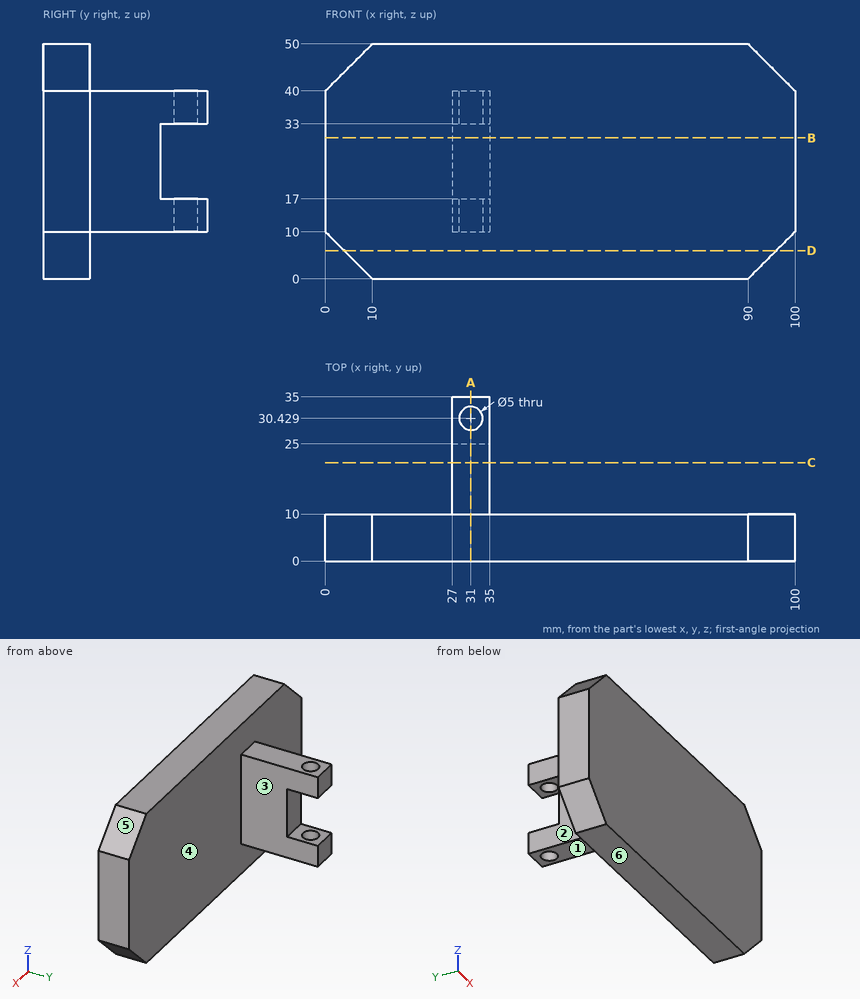
Drawing for the job (mm, zero at the part's lowest x, y, z). A direction names the side the tool comes from. Give positions to 0.01 mm unless a question says otherwise; leave off trailing zeros. Order: outer loops, then holes, each group sorted by start corner. A loop starts at its lowest first (then second) coordinate and runs counter-clockwise, first axis right, second up. Notation, with made-up numbers: M -33.5,70 L -5.5,70 A27 ccw -5.5,103 Z; hole C -28,23.25 d9. An arc over 180 degrees is marked long. Put each result on its own line as item: value. Start each with the question number.
(1) Saw through at A-A, the plane x = 31. Write the cut outline in (y, z).
(2) Saw through at D-D, the plane z = 6. Write the cut outline in (x, y).
(3) Saw through at C-C, the plane y = 21. Write the cut outline in (x, z).
(4) Mould opens along Z. For the marked faces 4, 5 and 6 say: +Z half, -Z half, draft (parallel to the pull), parting line (faces both ways), or undercut.
(5) Which spindle directions (+Z, -Z, +X, -X, +Y, -Y) get a long thin tool onto all of the face, cutting with end or side? Do the marked faces 1, 2 and 3. Say none if no direction does.
(6) Saw through at B-B, the plane z = 30. Write the cut outline in (x, y), then the cut area to 3 significant figures.
(7) Flat gauge pins, fed straight in: pin 1 Ø6 at (y, z) = (14, 37.5) entering from +X; pin 2 Ø6.5 at (x, y) = (30, 23.5) entering from -Z; pin 3 Ø9 at (x, y) = (32.5, 29) entering from +Z; pin 4 Ø5 at (y, z) = (16.5, 5.5) entering from +X. Where does each tip first touch, or does it go through?
(8) Drill centre lines: line 1 along Y through (x, z) = (31, 35); line 2 along X through (y, z) = (27, 14); line 3 along Z through (x, y) = (33, 19). Where is each one in solid material? Low to high.
Check result:
1. outline: M 0,0 L 10,0 L 10,10 L 27.93,10 L 27.93,17 L 25,17 L 25,33 L 27.93,33 L 27.93,40 L 10,40 L 10,50 L 0,50 Z; M 32.93,10 L 35,10 L 35,17 L 32.93,17 Z; M 32.93,33 L 35,33 L 35,40 L 32.93,40 Z
2. outline: M 4,0 L 96,0 L 96,10 L 4,10 Z
3. outline: M 27,10 L 35,10 L 35,40 L 27,40 Z
4. face 4: draft
4. face 5: +Z half
4. face 6: -Z half
5. face 1: -Z, +X, -X, +Y
5. face 2: +Z, -Z, -X, +Y
5. face 3: +Z, -Z, +X, +Y
6. outline: M 0,0 L 100,0 L 100,10 L 35,10 L 35,25 L 27,25 L 27,10 L 0,10 Z
6. area: 1,120 mm2
7. pin 1: stops at x = 35
7. pin 2: stops at z = 10
7. pin 3: stops at z = 40
7. pin 4: passes through
8. line 1: y = 0 to 27.93, 32.93 to 35
8. line 2: x = 27 to 35
8. line 3: z = 10 to 40
